Here's how the part is built. I have some questions about the finished solid (model axes, mm). Face numbers are marked on the shaded views. A direction names the side the tool comes from. Coordinates: 2 decimals unless noted, no trailing zeros. Write each loop counter-clockwise with the first axis right and the second up, starting at its lowest first coordinate (ties: lowest second). Pieces come first, ordered by that corner, then holes. Notation, with made-up numbers: M 46.5,12 L 101.5,12 A17 cw 101.5,31 Z; hole C 9.25,44 d1. An arc over 180 degrees is marked long. Use a Markdown table: item, result.
```python
from build123d import *

# Parameters (mm, degrees)
SKETCH_1_W          = 18
SKETCH_1_H          = 12
EXTRUDE_1_DEPTH     = 3
EXTRUDE_2_DEPTH     = 9
EXTRUDE1_DEPTH      = 18
SKETCH_5_R          = 1.5
CUT_EXTRUDE_5_DEPTH = 3
CHAMFER_1_SIZE      = 1
FILLET1_R           = 8
EXTRUDE6_REACH      = 51.295
EXTRUDE7_START      = -18
EXTRUDE7_DEPTH      = 18
FILLET5_R           = 3
FILLET6_R           = 5
FILLET7_R           = 8


with BuildPart() as part:
    # 草图1 → 拉伸1 (new body)
    with BuildSketch(Plane.XY):
        Rectangle(SKETCH_1_W, SKETCH_1_H)
    extrude(amount=EXTRUDE_1_DEPTH)

    # 草图2 → 拉伸2 (add, symmetric)
    with BuildSketch(Plane(origin=(0, 0, 0), x_dir=(0, 0, -1), z_dir=(1, 0, 0))):
        Polygon((19.392304845, 12), (45, 12), (45, 8.2), (20.665324997, 8.2), (0, 2.662742856), (-3, 6), align=None)
    extrude(amount=EXTRUDE_2_DEPTH, both=True)

    # Sketch2 → Extrude1 (add)
    with BuildSketch(Plane(origin=(9, 0, 0), x_dir=(0, 0, -1), z_dir=(1, 0, 0))):
        Polygon((45, 8.2), (20.665324997, 8.2), (14.65151871, 6.588605462), (20.665324997, -2), (45, -2), align=None)
    extrude(amount=-EXTRUDE1_DEPTH)

    # 草图5 → 拉伸5 (cut)
    with BuildSketch(Plane(origin=(0, 0, 0), x_dir=(-1, 0, 0), z_dir=(0, 0, -1))):
        with Locations((-5, -3)):
            Circle(SKETCH_5_R)
        with Locations((5, -3)):
            Circle(SKETCH_5_R)
    extrude(amount=-CUT_EXTRUDE_5_DEPTH, mode=Mode.SUBTRACT)

    # 倒角1
    chamfer_1_edges = [part.edges().sort_by_distance(p)[0] for p in [
        (9, -6, 1.5),
        (-9, -6, 1.5),
    ]]
    chamfer(chamfer_1_edges, length=CHAMFER_1_SIZE)

    # Fillet1
    fillet1_edges = [part.edges().sort_by_distance(p)[0] for p in [
        (0, 6, 3),
        (0, 12, -19.392304845),
    ]]
    fillet(fillet1_edges, radius=FILLET1_R)

    # Extrude6: up to this face of the body (flat: up to its plane)
    extrude6_end = Plane(part.part.faces().sort_by_distance((0, 12, -32.722762413))[0])
    # Sketch3 → Extrude6 (cut, up to the picked face)
    with BuildSketch(Plane.XZ.offset(6), mode=Mode.PRIVATE) as extrude6_sk1:
        with BuildLine():
            Line((-6, -45), (6, -45))
            Line((6, -45), (6, -13))
            ThreePointArc((6, -13), (0, -7), (-6, -13))
            Line((-6, -13), (-6, -45))
        make_face()
    extrude6_tool1 = split(extrude(extrude6_sk1.sketch, amount=-EXTRUDE6_REACH, mode=Mode.PRIVATE), bisect_by=extrude6_end, keep=Keep.BOTH, mode=Mode.PRIVATE)
    add(extrude6_tool1.solids().sort_by(Axis((0, -6, -26.619381), (0, 1, 0)))[0], mode=Mode.SUBTRACT)

    # Sketch4 → Extrude7 (cut)
    with BuildSketch(Plane(origin=(9, 0, 0), x_dir=(0, 0, -1), z_dir=(1, 0, 0)).offset(EXTRUDE7_START)):
        with BuildLine():
            Line((26, 8.6), (45, 8.6))
            Line((45, 8.6), (45, 1.4))
            Line((45, 1.4), (26, 1.4))
            ThreePointArc((26, 1.4), (22.4, 5), (26, 8.6))
        make_face()
    extrude(amount=EXTRUDE7_DEPTH, mode=Mode.SUBTRACT)

    # Fillet5
    fillet5_edges = [part.edges().sort_by_distance(p)[0] for p in [
        (0, 2.662742856, 0),
    ]]
    fillet(fillet5_edges, radius=FILLET5_R)

    # Fillet6
    fillet6_edges = [part.edges().sort_by_distance(p)[0] for p in [
        (-7.5, 6.588605462, -14.65151871),
        (7.5, 6.588605462, -14.65151871),
    ]]
    fillet(fillet6_edges, radius=FILLET6_R)

    # Fillet7
    fillet7_edges = [part.edges().sort_by_distance(p)[0] for p in [
        (-7.5, -2, -20.665324997),
        (7.5, -2, -20.665324997),
    ]]
    fillet(fillet7_edges, radius=FILLET7_R)


solid = part.part
```
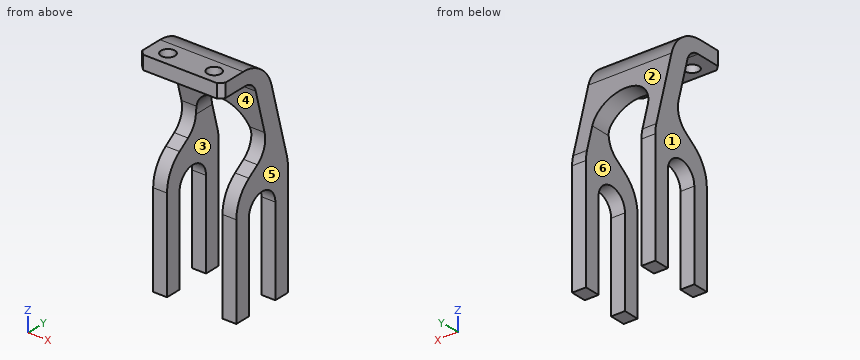
1. Suppose I cut it at C-C on z = -16. Write out the boundary of the cut face in (x, y), and give its area (3 significant figures).
Answers follow:
| item | result |
|---|---|
| outline | M -9,4.49 L -6,4.49 L -6,11.09 L -9,11.09 Z; M 6,4.49 L 9,4.49 L 9,11.09 L 6,11.09 Z |
| area | 39.6 mm2 |
2. We'd pull the mould along X, two halves only. Please class the marked faces 1, 2 and 3: +X half, -X half, draft (parallel to the pull), parting line (faces both ways), or undercut.
Answers follow:
| item | result |
|---|---|
| face 1 | -X half |
| face 2 | draft |
| face 3 | undercut |
3. I need wall thicknesses on probe 1 along Y at (x, z) = (8.25, -31); probe 2 along X at (y, z) = (11, -35); probe 3 along Z at (x, y) = (4.5, -5). Which ranges of each line are inside material? Lowest first, please.
Answers follow:
| item | result |
|---|---|
| probe 1 | y = -2 to 1.4, 8.6 to 12 |
| probe 2 | x = -9 to -6, 6 to 9 |
| probe 3 | z = 0 to 3 |
4. Suppose I cut it at D-D on x = -5. Write out the boundary of the cut face in (y, z), and give its area (3 significant figures).
Answers follow:
| item | result |
|---|---|
| outline | M -6,0 L -4.5,0 L -4.5,3 L -6,3 Z; M -1.5,0 L 0.36,0 A3 cw 3.26,-2.22 L 5.26,-9.68 L 9.4,-9.68 L 7.59,-2.93 A8 ccw -0.14,3 L -1.5,3 Z |
| area | 62.1 mm2 |
5. Will these pins go through, and if not, where does the flat tip stop? pin 1 Ø1 at (x, y) = (2, 5) entering from +Z; pin 2 Ø0.9 at (x, z) = (-7.5, -35) entering from -Y; pin 3 Ø1 at (x, y) = (-4, 2) entering from +Z; pin 4 Ø5 at (x, y) = (5, -3) entering from +Z.
Answers follow:
| item | result |
|---|---|
| pin 1 | stops at z = 1.52 |
| pin 2 | stops at y = -2 |
| pin 3 | stops at z = 2.83 |
| pin 4 | stops at z = 3 |
6. Suppose I cut it at B-B on x = 4.5. Write out the boundary of the cut face in (y, z).
Answers follow:
| item | result |
|---|---|
| outline | M -6,0 L -4.41,0 L -4.41,3 L -6,3 Z; M -1.59,0 L 0.36,0 A3 cw 3.26,-2.22 L 5.08,-9.03 L 9.22,-9.03 L 7.59,-2.93 A8 ccw -0.14,3 L -1.59,3 Z |
7. Suppose I cut it at A-A on z = -27.5. Write out the boundary of the cut face in (x, y).
Answers follow:
| item | result |
|---|---|
| outline | M -9,-2 L -6,-2 L -6,1.4 L -9,1.4 Z; M -9,8.6 L -6,8.6 L -6,12 L -9,12 Z; M 6,-2 L 9,-2 L 9,1.4 L 6,1.4 Z; M 6,8.6 L 9,8.6 L 9,12 L 6,12 Z |
8. Which directions (+Z, -Z, +X, -X, +Y, -Y) give clear straight access to the entire face, cutting with the end or side of a thin tool? Please do the marked faces 4, 5 and 6.
Answers follow:
| item | result |
|---|---|
| face 4 | +X, -X, -Y |
| face 5 | +Z, -Z, +X, +Y, -Y |
| face 6 | -Z, +Y, -Y |
